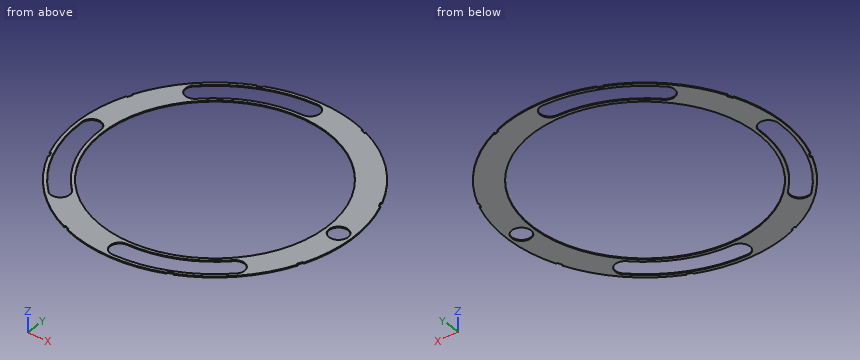
```python
from build123d import *

# Parameters (mm, degrees)
SKETCH4_R           = 68.072
BOSS_EXTRUDE2_DEPTH = 0.508
SKETCH5_R           = 55.372
CUT_EXTRUDE5_DEPTH  = 1.508
SKETCH6_R           = 4.699
CUT_EXTRUDE6_DEPTH  = 1.508
CUT_EXTRUDE11_DEPTH = 1.508


with BuildPart() as part:
    # Sketch4 → Boss-Extrude2 (new body)
    with BuildSketch(Plane.XY):
        Circle(SKETCH4_R)
    extrude(amount=BOSS_EXTRUDE2_DEPTH)

    # Sketch5 → Cut-Extrude5 (cut, through all)
    with BuildSketch(Plane.XY.offset(0.508)):
        Circle(SKETCH5_R)
    extrude(amount=-CUT_EXTRUDE5_DEPTH, mode=Mode.SUBTRACT)

    # Sketch6 → Cut-Extrude6 (cut, through all)
    with BuildSketch(Plane.XY.offset(0.508)):
        with Locations((61.722, 0)):
            Circle(SKETCH6_R)
        with BuildLine():
            ThreePointArc((46.966739403, -46.966739623), (46.966739521, -40.321349991), (40.321349889, -40.321350078))
            ThreePointArc((40.321349889, -40.321350078), (21.821757973, -52.68238233), (1.451e-06, -57.023))
            ThreePointArc((1.451e-06, -57.023), (-4.699, -61.72200012), (1.691e-06, -66.421))
            ThreePointArc((1.691e-06, -66.421), (25.41821697, -61.365002135), (46.966739403, -46.966739623))
        make_face()
        with BuildLine():
            ThreePointArc((-46.966739623, -46.966739403), (-40.321349991, -46.966739521), (-40.321350078, -40.321349889))
            ThreePointArc((-40.321350078, -40.321349889), (-52.68238233, -21.821757973), (-57.023, -1.451e-06))
            ThreePointArc((-57.023, -1.451e-06), (-61.72200012, 4.699), (-66.421, -1.69e-06))
            ThreePointArc((-66.421, -1.69e-06), (-61.365002135, -25.41821697), (-46.966739623, -46.966739403))
        make_face()
        with BuildLine():
            ThreePointArc((-46.966739403, 46.966739623), (-46.966739521, 40.321349991), (-40.321349889, 40.321350078))
            ThreePointArc((-40.321349889, 40.321350078), (-21.821757973, 52.68238233), (-1.451e-06, 57.023))
            ThreePointArc((-1.451e-06, 57.023), (4.699, 61.72200012), (-1.69e-06, 66.421))
            ThreePointArc((-1.69e-06, 66.421), (-25.41821697, 61.365002135), (-46.966739403, 46.966739623))
        make_face()
    extrude(amount=-CUT_EXTRUDE6_DEPTH, mode=Mode.SUBTRACT)

    # Sketch8 → Cut-Extrude11 (cut, through all)
    with BuildSketch(Plane.XY.offset(0.508)):
        Polygon((63.962998999, 25.119703581), (62.990983081, 27.466357594), (61.817656075, 26.980349635), (62.789671993, 24.633695622), align=None)
        Polygon((-25.119703581, 63.962998999), (-27.466357594, 62.990983081), (-26.980349635, 61.817656075), (-24.633695622, 62.789671993), align=None)
        Polygon((-62.990983081, 27.466357594), (-63.962998999, 25.119703581), (-62.789671993, 24.633695622), (-61.817656075, 26.980349635), align=None)
        Polygon((-63.962998999, -25.119703581), (-62.990983081, -27.466357594), (-61.817656075, -26.980349635), (-62.789671993, -24.633695622), align=None)
        Polygon((-27.466357594, -62.990983081), (-25.119703581, -63.962998999), (-24.633695622, -62.789671993), (-26.980349635, -61.817656075), align=None)
        Polygon((25.119703581, -63.962998999), (27.466357594, -62.990983081), (26.980349635, -61.817656075), (24.633695622, -62.789671993), align=None)
        Polygon((62.990983081, -27.466357594), (63.962998999, -25.119703581), (62.789671993, -24.633695622), (61.817656075, -26.980349635), align=None)
        Polygon((27.466357594, 62.990983081), (25.119703581, 63.962998999), (24.633695622, 62.789671993), (26.980349635, 61.817656075), align=None)
    extrude(amount=-CUT_EXTRUDE11_DEPTH, mode=Mode.SUBTRACT)


solid = part.part
```
Verification items for the finished model (mm, model axes). Coordinates: 2 decimals unless noted, no trailing zeros. Order: outer loops, then holes, each group sorted by start corner. A loop starts at its lowest first (then second) coordinate and runs counter-clockwise, first axis right, second up. Notation, with made-up numbers: (0, -25) -> (24, -25) arc R21 ccw to (24, 8) -> close; hole circle Ø1 at (-14.75, 25.25). An arc over 180 degrees is marked (long way). Put each result on its own line as item: value. Start each with the question number.
1) Cross-section at C-C (z = 0.25). State how many separate pieces and enclosed holes the cut face has, plus the area to 3 significant figures.
2) Cross-section at D-D (x = 20). Enter the section's corners in (y, z), plus the area to 3 significant figures.
3) Cross-section at B-B (x = -44.5). Enter the section's corners in (y, z).
4) Cross-section at A-A (y = -13.5). Enter the section's corners in (x, z).
5) Material ranges on L1, parallel to Y at x = 43.5, z = 0.15; L2, parallel to X at y = 3.5, z = 0.1; L3, parallel to X at y = -1, z = 0.35, recorded low to high.
Geometry check:
1. separate pieces: 1
1. enclosed holes: 5
1. area: 3,270 mm^2
2. outline: (-65.07, 0) -> (-63.34, 0) -> (-63.34, 0.51) -> (-65.07, 0.51) -> close; (-53.4, 0) -> (-51.63, 0) -> (-51.63, 0.51) -> (-53.4, 0.51) -> close; (51.63, 0) -> (65.07, 0) -> (65.07, 0.51) -> (51.63, 0.51) -> close
2. area: 8.60 mm^2
3. outline: (-51.51, 0) -> (-48.26, 0) -> (-48.26, 0.51) -> (-51.51, 0.51) -> close; (-35.66, 0) -> (-32.95, 0) -> (-32.95, 0.51) -> (-35.66, 0.51) -> close; (32.95, 0) -> (39.02, 0) -> (39.02, 0.51) -> (32.95, 0.51) -> close; (49.31, 0) -> (51.51, 0) -> (51.51, 0.51) -> (49.31, 0.51) -> close
4. outline: (-66.72, 0) -> (-65.03, 0) -> (-65.03, 0.51) -> (-66.72, 0.51) -> close; (-55.4, 0) -> (-53.7, 0) -> (-53.7, 0.51) -> (-55.4, 0.51) -> close; (53.7, 0) -> (66.72, 0) -> (66.72, 0.51) -> (53.7, 0.51) -> close
5. L1: y = -52.36 to -50.19, -38.95 to -34.26, 34.26 to 52.36
5. L2: x = -67.98 to -64.86, -58.59 to -55.26, 55.26 to 58.59, 64.86 to 67.98
5. L3: x = -68.06 to -66.41, -57.01 to -55.36, 55.36 to 57.13, 66.31 to 68.06
